from build123d import *

# Parameters (mm, degrees)
F2_R     = 52.5
F2_R_2   = 40
F3_DEPTH = 2
F4_R     = 9
F5_DEPTH = 5
F7_DEPTH = 10
F9_DEPTH = 6


with BuildPart() as f1:
    # F0 (on Front) → F1 (revolve)
    with BuildSketch(Plane.XZ):
        Polygon((-73, 0), (0, 0), (0, 5), (-69.75, 5), (-69.75, 6), (-71.25, 6), (-71.25, 5), (-73, 5), align=None)
    revolve(axis=Axis((0, 0, 2.5), (0, 0, -1)))

    # F2 (on face) → F3 (cut)
    with BuildSketch(Plane(origin=(0, 0, 0), x_dir=(1, 0, 0), z_dir=(0, 0, -1))):
        Circle(F2_R)
        Circle(F2_R_2, mode=Mode.SUBTRACT)
    extrude(amount=-F3_DEPTH, mode=Mode.SUBTRACT)

    # F4 (on face) → F5 (cut, through all)
    with BuildSketch(Plane.XY.offset(5)):
        Circle(F4_R)
    extrude(amount=-F5_DEPTH, mode=Mode.SUBTRACT)

    # F6 (on face) → F7 (join)
    with BuildSketch(Plane.XY.offset(5)):
        with BuildLine():
            ThreePointArc((59.75, -2.5), (59.802278, 0), (59.75, 2.5))
            Line((59.75, 2.5), (54.75, 2.5))
            ThreePointArc((54.75, 2.5), (54.807048, 0), (54.75, -2.5))
            Line((54.75, -2.5), (59.75, -2.5))
        make_face()
        with BuildLine():
            ThreePointArc((-29.540064, 46.164891), (-27.403524, 47.464296), (-25.209936, 48.664891))
            Line((-25.209936, 48.664891), (-27.709936, 52.995018))
            ThreePointArc((-27.709936, 52.995018), (-29.901139, 51.790292), (-32.040064, 50.495018))
            Line((-32.040064, 50.495018), (-29.540064, 46.164891))
        make_face()
        with BuildLine():
            ThreePointArc((-25.209936, -48.664891), (-27.403524, -47.464296), (-29.540064, -46.164891))
            Line((-29.540064, -46.164891), (-32.040064, -50.495018))
            ThreePointArc((-32.040064, -50.495018), (-29.901139, -51.790292), (-27.709936, -52.995018))
            Line((-27.709936, -52.995018), (-25.209936, -48.664891))
        make_face()
    extrude(amount=F7_DEPTH)

    # F8 (on face) → F9 (cut, through all)
    with BuildSketch(Plane.XY.offset(6)):
        with BuildLine():
            Line((-49.426388, 42.214123), (-55.509635, 47.409708))
            ThreePointArc((-55.509635, 47.409708), (-73, 0), (-55.509635, -47.409708))
            Line((-55.509635, -47.409708), (-49.426388, -42.214123))
            ThreePointArc((-49.426388, -42.214123), (-65, 0), (-49.426388, 42.214123))
        make_face()
    extrude(amount=-F9_DEPTH, mode=Mode.SUBTRACT)


solid = f1.part
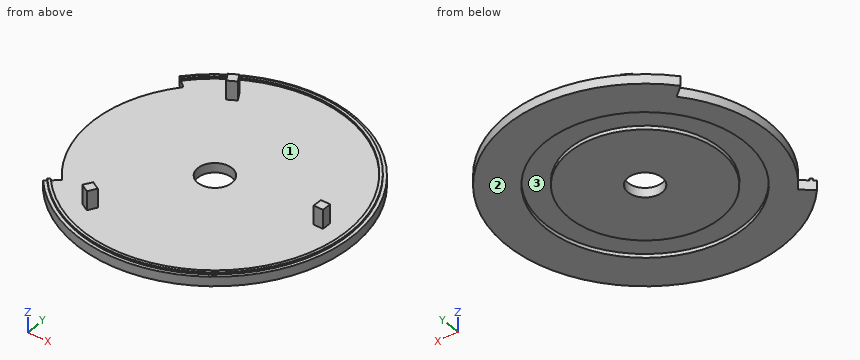
Check sheet for the modelled part. Datum: model origin and axes. Units: mm. Face numbers are marked on the shaded views. Give positions to 0.01 mm unless a question says otherwise; leave off trailing zeros. Write each loop counter-clockwise with the first axis right and the second up, starting at its lowest first coordinate (ties: lowest second). Pieces come first, ordered by that corner, then holes. Notation, with made-up numbers: M 80,21 L 91,21 A30 cw 91,57 Z; hole C -10,21 d11. An arc over 180 degrees is marked long. Use one line per item in the form item = value.
(1) Section check B-B on y = 0. Record the boundary of the cut face in (x, z), plus the area to 3 significant figures.
Answer block:
outline = M -65,0 L -52.5,0 L -52.5,2 L -40,2 L -40,0 L -9,0 L -9,5 L -65,5 Z; M 9,0 L 40,0 L 40,2 L 52.5,2 L 52.5,0 L 73,0 L 73,5 L 71.25,5 L 71.25,6 L 69.75,6 L 69.75,5 L 59.8,5 L 59.8,15 L 54.81,15 L 54.81,5 L 9,5 Z
area = 601 mm2
(2) Section check C-C on x = 0. Record the boundary of the cut face in (y, z), plus the area to 3 significant figures.
Answer block:
outline = M -73,0 L -52.5,0 L -52.5,2 L -40,2 L -40,0 L -9,0 L -9,5 L -69.75,5 L -69.75,6 L -71.25,6 L -71.25,5 L -73,5 Z; M 9,0 L 40,0 L 40,2 L 52.5,2 L 52.5,0 L 73,0 L 73,5 L 71.25,5 L 71.25,6 L 69.75,6 L 69.75,5 L 9,5 Z
area = 593 mm2
(3) Material ranges on line 1 along Y through (x, z) = (0, 2.15); line 2 along X through (y, z) = (0, 5.8); line 3 along Y through (x, z) = (0, 5.7), recorded low to high.
Answer block:
line_1 = -73 to -9, 9 to 73
line_2 = 54.81 to 59.8, 69.75 to 71.25
line_3 = -71.25 to -69.75, 69.75 to 71.25
(4) Depth check by flat-ended pin: P1, Ø1.5, axis at x = 56.5, z = 9.5, coming from the +Y side; P2, Ø5.5, axis at x = 56, z = 10, coming from the -Y side; P3, Ø8, axis at y = 5.5, z = 8.5, coming from the +X side. Enter the tip coordinate at first touch or a pass-through.
Answer block:
P1 = 2.5
P2 = -2.5
P3 = 72.91
(5) Section check A-A on z = 11. Record the boundary of the cut face in (x, y), plus the area to 3 significant figures.
Answer block:
outline = M -32.04,-50.5 A59.8 ccw -27.71,-53 L -25.21,-48.66 A54.81 cw -29.54,-46.16 Z; M -32.04,50.5 L -29.54,46.16 A54.81 cw -25.21,48.66 L -27.71,53 A59.8 ccw Z; M 54.75,-2.5 L 59.75,-2.5 A59.8 ccw 59.75,2.5 L 54.75,2.5 A54.81 cw Z
area = 75.0 mm2
(6) Section check D-D on x = -46.5. Record the boundary of the cut face in (y, z), plus the area to 3 significant figures.
Answer block:
outline = M -56.27,0 L -24.37,0 L -24.37,2 L 24.37,2 L 24.37,0 L 56.27,0 L 56.27,5 L 53.98,5 L 53.98,6 L 51.99,6 L 51.99,5 L -51.99,5 L -51.99,6 L -53.98,6 L -53.98,5 L -56.27,5 Z
area = 469 mm2
(7) Draft check along X on the marked faces 1, 2 and 3. Enter one of: pulls with the +X half, pulls with the -X half, needs draft (parallel to the pull), parting line crosses it, or undercut.
Answer block:
face_1 = undercut
face_2 = needs draft
face_3 = undercut
